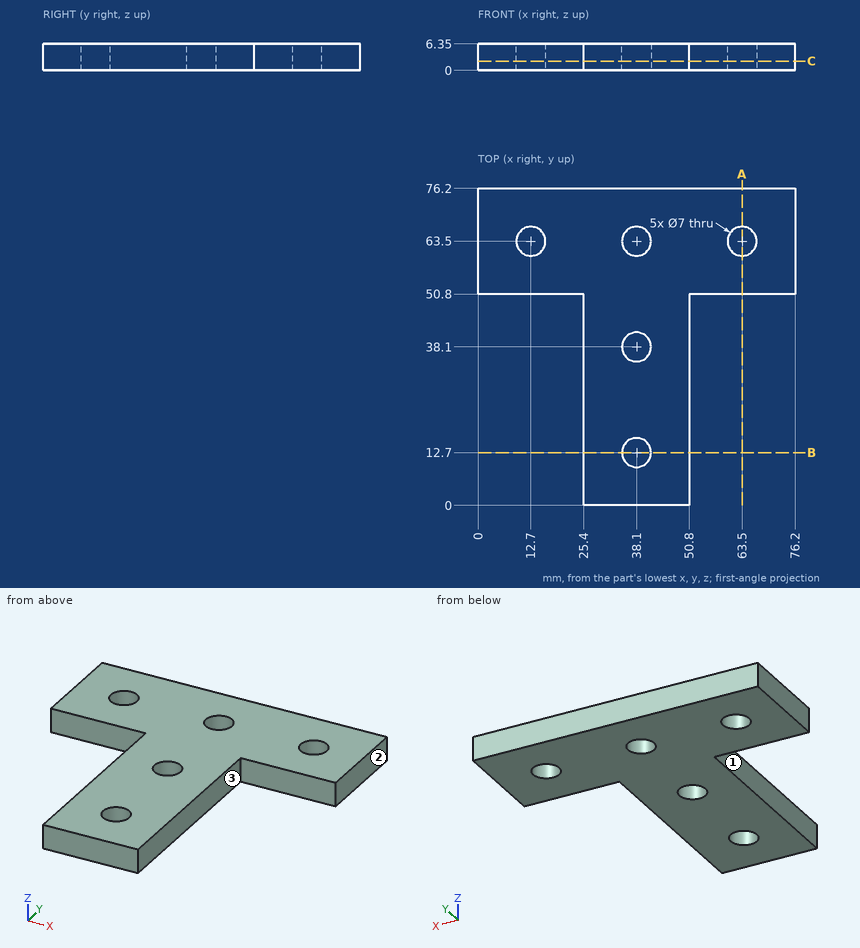
Can you work these out from the drawing? Everything is in mm from the part's minimum corner. A direction names the side the tool comes from. Coordinates: 2 decimals unless noted, no trailing zeros. Loops run counter-clockwise (first coordinate to the right, second up) from the corner with the lowest first, then second, coordinate; pieces in that order, holes last.
1) Imagine slicing it at A-A on x = 63.5. List the corners of the cut face in (y, z) for me, plus the area to 3 significant figures.
2) For pin 1 (11 mm diameter, centred on x = 12.7, y = 63.5, fed in from +Z); pin 2 (1.9 mm diameter, centred on x = 9, z = 2, fed in from -Y); pin 3 (1 mm diameter, centred on y = 26, z = 5.5, fed in from +X); pin 4 (1 mm diameter, centred on y = 12, z = 1.5, fed in from -X), each with a flat end and sliding along its axis, tell me the tip position at first contact or that it passes through.
3) Which directions (+Z, -Z, +X, -X, +Y, -Y) give clear straight access to the entire face, cutting with the end or side of a thin tool? Please do the marked faces 1, 2 and 3.
4) I need wall thicknesses on probe 1 along Y at (x, z) = (38.1, 1.75); probe 2 along Y at (x, z) = (63.5, 1.75); probe 3 along X at (y, z) = (62, 0.5). Which ranges of each line are inside material? Lowest first, please.
5) Imagine slicing it at C-C on z = 2.25. List the corners of the cut face in (x, y) for me, plus the area to 3 significant figures.
6) Imagine slicing it at B-B on y = 12.7. List the corners of the cut face in (x, z) for me, plus the area to 3 significant figures.
Completed:
1. outline: (50.8, 0) - (60, 0) - (60, 6.35) - (50.8, 6.35) - close; (67, 0) - (76.2, 0) - (76.2, 6.35) - (67, 6.35) - close
1. area: 117 mm2
2. pin 1: stops at z = 6.35
2. pin 2: stops at y = 50.8
2. pin 3: stops at x = 50.8
2. pin 4: stops at x = 25.4
3. face 1: +Z, -Z, -X, -Y
3. face 2: +Z, -Z, +X, +Y, -Y
3. face 3: +Z, -Z, +X, -Y
4. probe 1: y = 0 to 9.2, 16.2 to 34.6, 41.6 to 60, 67 to 76.2
4. probe 2: y = 50.8 to 60, 67 to 76.2
4. probe 3: x = 0 to 9.54, 15.86 to 34.94, 41.26 to 60.34, 66.66 to 76.2
5. outline: (0, 50.8) - (25.4, 50.8) - (25.4, 0) - (50.8, 0) - (50.8, 50.8) - (76.2, 50.8) - (76.2, 76.2) - (0, 76.2) - close; hole circle Ø7 at (12.7, 63.5); hole circle Ø7 at (38.1, 12.7); hole circle Ø7 at (38.1, 38.1); hole circle Ø7 at (38.1, 63.5); hole circle Ø7 at (63.5, 63.5)
5. area: 3,030 mm2
6. outline: (25.4, 0) - (34.6, 0) - (34.6, 6.35) - (25.4, 6.35) - close; (41.6, 0) - (50.8, 0) - (50.8, 6.35) - (41.6, 6.35) - close
6. area: 117 mm2
